```python
from build123d import *

# Parameters (mm, degrees)
SKETCH1_W           = 66.7
SKETCH1_H           = 288.29
SKETCH1_R           = 1.3890625
SKETCH1_R_2         = 1.7859375
SKETCH1_R_3         = 2.54
SKETCH1_R_4         = 12.7
SKETCH1_W_2         = 5.08
SKETCH1_H_2         = 5.08
SKETCH1_W_3         = 26
SKETCH1_H_3         = 72
BOSS_EXTRUDE1_DEPTH = 6.35


with BuildPart() as part:
    # Sketch1 → Boss-Extrude1 (new body)
    with BuildSketch(Plane.XY):
        with Locations((33.35, -144.145)):
            Rectangle(SKETCH1_W, SKETCH1_H)
        with Locations((63.16, -269.875)):
            Circle(SKETCH1_R, mode=Mode.SUBTRACT)
        with Locations((63.16, -250.825)):
            Circle(SKETCH1_R, mode=Mode.SUBTRACT)
        with Locations((15.54, -250.825)):
            Circle(SKETCH1_R, mode=Mode.SUBTRACT)
        with Locations((15.54, -269.875)):
            Circle(SKETCH1_R, mode=Mode.SUBTRACT)
        with Locations((55.675, -133.39)):
            Circle(SKETCH1_R_2, mode=Mode.SUBTRACT)
        with Locations((55.675, -189.39)):
            Circle(SKETCH1_R_2, mode=Mode.SUBTRACT)
        with Locations((33.35, -88.85)):
            Circle(SKETCH1_R_3, mode=Mode.SUBTRACT)
        with Locations((33.35, -47.6)):
            Circle(SKETCH1_R_4, mode=Mode.SUBTRACT)
        with Locations((33.35, -6.35)):
            Circle(SKETCH1_R_3, mode=Mode.SUBTRACT)
        with Locations((63.16, -260.35)):
            Rectangle(SKETCH1_W_2, SKETCH1_H_2, mode=Mode.SUBTRACT)
        with Locations((15.54, -260.35)):
            Rectangle(SKETCH1_W_2, SKETCH1_H_2, mode=Mode.SUBTRACT)
        with Locations((37.05, -154.29)):
            Rectangle(SKETCH1_W_3, SKETCH1_H_3, mode=Mode.SUBTRACT)
    extrude(amount=BOSS_EXTRUDE1_DEPTH)


solid = part.part
```
Design review of the part built by this model. Coordinates are the model's own, in mm. A direction names the side the tool comes from. Give positions to 0.01 mm unless a question says otherwise; leave off trailing zeros. Loops run counter-clockwise (first coordinate to the right, second up) from the corner with the lowest first, then second, coordinate; pieces in that order, holes last. Notation, with made-up numbers: M -17,4.5 L 19,4.5 A28 cw 19,33.5 Z; hole C 16.25,77.25 d4. An arc over 180 degrees is marked long. Return JSON: item names as keys, results as strings. Group by question number.
Item 1: Tool access review of faces 4 (the flat face through (37, -190.29, 3)), 5 (the flat face through (18, -142, 0)): name each direction out of +Z, -Z, +X, -X, +Y, -Y from which nothing blocks a thin tool from reaching the whole face with its end or side.
Item 2: We need section B-B (y = -47.6). Give the boundary of the cut face in (x, z).
Item 3: Mouldability with a two-part tool opening along X and no side actions: class faces 1 (the flat face through (0, -146, 3)), 2 (the flat face through (63, -257.81, 3)), 3 (the flat face through (33, 0, 3)) as released by +X, released by -X, zero draft, split by the parting line, or undercut.
Item 4: We need section C-C (z = 4.25). Give the number of separate pieces and of enclosed holes in the cut face, and give its area (3 significant figures).
Item 5: We need section D-D (y = -6.35). Give the boundary of the cut face in (x, z), and give its area (3 significant figures).
Item 6: For probe 1 along X at (y, z) = (-259, 2); probe 2 along Y at (x, z) = (33.35, 2); probe 3 along Y at (x, z) = (63.16, 1.5), list the stretches that pass through material, from the lowest coordinate up.
Item 7: We need section A-A (x = 33.35). Give the boundary of the cut face in (y, z).
Item 8: Insertion check: pin 1 Ø2.5 at (x, y) = (15.54, -250.825) entering from -Z. The pin has a flat end and moves straight along its axis. Give the tip position at first contact, or say it passes through.
Output:
{
 "1": {"face 4": "+Z, -Z", "face 5": "-Z, +X, -X, +Y, -Y"},
 "2": {"outline": "M 0,0 L 20.65,0 L 20.65,6.35 L 0,6.35 Z; M 46.05,0 L 66.7,0 L 66.7,6.35 L 46.05,6.35 Z"},
 "3": {"face 1": "released by -X", "face 2": "undercut", "face 3": "zero draft"},
 "4": {"separate pieces": "1", "enclosed holes": "12", "area": "16,700 mm^2"},
 "5": {"outline": "M 0,0 L 30.81,0 L 30.81,6.35 L 0,6.35 Z; M 35.89,0 L 66.7,0 L 66.7,6.35 L 35.89,6.35 Z", "area": "391 mm^2"},
 "6": {"probe 1": "x = 0 to 13, 18.08 to 60.62, 65.7 to 66.7", "probe 2": "y = -288.29 to -190.29, -118.29 to -91.39, -86.31 to -60.3, -34.9 to -8.89, -3.81 to 0", "probe 3": "y = -288.29 to -271.26, -268.49 to -262.89, -257.81 to -252.21, -249.44 to 0"},
 "7": {"outline": "M -288.29,0 L -190.29,0 L -190.29,6.35 L -288.29,6.35 Z; M -118.29,0 L -91.39,0 L -91.39,6.35 L -118.29,6.35 Z; M -86.31,0 L -60.3,0 L -60.3,6.35 L -86.31,6.35 Z; M -34.9,0 L -8.89,0 L -8.89,6.35 L -34.9,6.35 Z; M -3.81,0 L 0,0 L 0,6.35 L -3.81,6.35 Z"},
 "8": {"pin 1": "passes through"}
}
